The figure shows three views and two pictorial views of one solid part (mm, origin at its lowest corner). Answer the questions. Give positions to 0.01 mm unless a question says otherwise; leave off trailing zeros. Loops run counter-clockwise (first coordinate to the right, second up) from the corner with the lowest first, then second, coordinate; pieces in that order, holes last. Notation, with made-up numbers: (68.5, 19) - (111.5, 19) arc R26 ccw to (111.5, 39) - close; hole circle Ø2 at (26, 83.5). An arc over 180 degrees is marked (long way). Use CSV: the item, a comma, the result in double quotes.
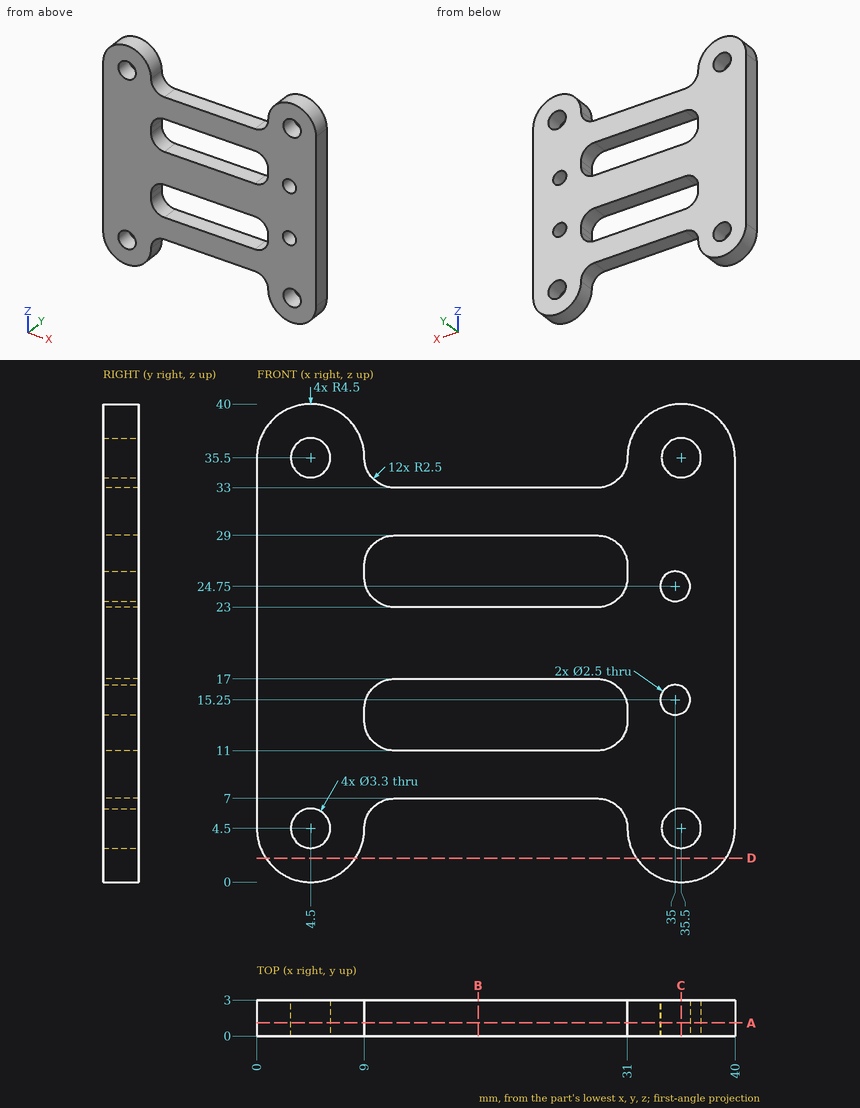
Item 1: Given P1, Ø2, axis at x = 35, z = 15.25, coming from the -Y side; P2, Ø0.9, axis at x = 18, y = 1, coming from the +Z side, each flat-ended and moving along its own axis, determine where each tip first touches the part or whether it passes through.
Determined:
P1,"passes through"
P2,"stops at z = 33"
Item 2: A cutting plane is placed at B-B on x = 18.5. Determine the outline of the cut face in (y, z), and give its area (3 significant figures).
Determined:
outline,"(0, 7) - (3, 7) - (3, 11) - (0, 11) - close; (0, 17) - (3, 17) - (3, 23) - (0, 23) - close; (0, 29) - (3, 29) - (3, 33) - (0, 33) - close"
area,"42.0 mm²"
Item 3: A cutting plane is placed at D-D on z = 2. Determine the outline of the cut face in (x, y).
Determined:
outline,"(0.76, 0) - (8.24, 0) - (8.24, 3) - (0.76, 3) - close; (31.76, 0) - (39.24, 0) - (39.24, 3) - (31.76, 3) - close"
Item 4: A cutting plane is placed at A-A on y = 1.1. State how many separate pieces and enclosed holes the cut face has, and give its area (3 significant figures).
Determined:
separate pieces,"1"
enclosed holes,"8"
area,"965 mm²"
Item 5: Find the intervals of material crossed by line 1 (Z direction, x = 24.5, y = 2.55); line 2 (Z direction, x = 11, y = 2.75); line 3 (Z direction, x = 35, y = 2.3), in increasing order.
Determined:
line 1,"z = 7 to 11, 17 to 23, 29 to 33"
line 2,"z = 6.95 to 11.05, 16.95 to 23.05, 28.95 to 33.05"
line 3,"z = 0.03 to 2.93, 6.07 to 14, 16.5 to 23.5, 26 to 33.93, 37.07 to 39.97"
Item 6: A cutting plane is placed at C-C on x = 35.5. Determine the outline of the cut face in (y, z), and give its area (3 significant figures).
Determined:
outline,"(0, 0) - (3, 0) - (3, 2.85) - (0, 2.85) - close; (0, 6.15) - (3, 6.15) - (3, 14.1) - (0, 14.1) - close; (0, 16.4) - (3, 16.4) - (3, 23.6) - (0, 23.6) - close; (0, 25.9) - (3, 25.9) - (3, 33.85) - (0, 33.85) - close; (0, 37.15) - (3, 37.15) - (3, 40) - (0, 40) - close"
area,"86.5 mm²"
